Geometry check sheet. Reference: the model listing, model coordinates, mm. A direction names the side the tool comes from. Coordinates: 2 decimals unless noted, no trailing zeros. Write each loop counter-clockwise with the first axis right and the second up, starting at its lowest first coordinate (ties: lowest second). Pieces come first, ordered by that corner, then holes.
from build123d import *

# Parameters (mm, degrees)
SKETCH1_W           = 29
SKETCH1_H           = 15.5
BOSS_EXTRUDE1_DEPTH = 8
SHELL1_T            = -1
SKETCH2_W           = 1
SKETCH2_H           = 13.5
BOSS_EXTRUDE2_DEPTH = 7
SKETCH3_W           = 8
SKETCH3_H           = 3
CUT_EXTRUDE1_DEPTH  = 7


with BuildPart() as part:
    # Sketch1 → Boss-Extrude1 (new body)
    with BuildSketch(Plane(origin=(0, 0, 0), x_dir=(1, 0, 0), z_dir=(0, 1, 0))):
        Rectangle(SKETCH1_W, SKETCH1_H)
    extrude(amount=BOSS_EXTRUDE1_DEPTH)

    # Shell1
    shell1_openings = [part.faces().sort_by_distance(p)[0] for p in [
        (0, 8, 0),
    ]]
    offset(amount=SHELL1_T, openings=shell1_openings, kind=Kind.INTERSECTION)

    # Sketch2 → Boss-Extrude2 (add)
    with BuildSketch(Plane(origin=(0, 1, 0), x_dir=(1, 0, 0), z_dir=(0, 1, 0))):
        Rectangle(SKETCH2_W, SKETCH2_H)
    extrude(amount=BOSS_EXTRUDE2_DEPTH)

    # Sketch3 → Cut-Extrude1 (cut)
    with BuildSketch(Plane(origin=(0, 1, 0), x_dir=(1, 0, 0), z_dir=(0, 1, 0))):
        with Locations((-7.25, 5.25)):
            Rectangle(SKETCH3_W, SKETCH3_H)
        with Locations((7.25, 5.25)):
            Rectangle(SKETCH3_W, SKETCH3_H)
        with Locations((7.25, -5.25)):
            Rectangle(SKETCH3_W, SKETCH3_H)
        with Locations((-7.25, -5.25)):
            Rectangle(SKETCH3_W, SKETCH3_H)
    extrude(amount=-CUT_EXTRUDE1_DEPTH, mode=Mode.SUBTRACT)


solid = part.part
1. Sectioned sample at A-A, the plane x = -9.5. Record the boundary of the cut face in (y, z), and give its area (3 significant figures).
Computed values:
outline: (0, -7.75) - (8, -7.75) - (8, -6.75) - (0, -6.75) - close; (0, -3.75) - (1, -3.75) - (1, 3.75) - (0, 3.75) - close; (0, 6.75) - (8, 6.75) - (8, 7.75) - (0, 7.75) - close
area: 23.5 mm2
2. Thickness scan on line 1 along X through (y, z) = (5.75, -3.5); line 2 along Z through (x, y) = (8.5, 0.5); line 3 along Z through (x, y) = (-5, 5.5). Record the ranges inside material, lowest first.
Computed values:
line 1: x = -14.5 to -13.5, -0.5 to 0.5, 13.5 to 14.5
line 2: z = -7.75 to -6.75, -3.75 to 3.75, 6.75 to 7.75
line 3: z = -7.75 to -6.75, 6.75 to 7.75
3. Sectioned sample at B-B, the plane z = 5.75. Record the boundary of the cut face in (x, y).
Computed values:
outline: (-14.5, 0) - (-11.25, 0) - (-11.25, 1) - (-13.5, 1) - (-13.5, 8) - (-14.5, 8) - close; (-3.25, 0) - (3.25, 0) - (3.25, 1) - (0.5, 1) - (0.5, 8) - (-0.5, 8) - (-0.5, 1) - (-3.25, 1) - close; (11.25, 0) - (14.5, 0) - (14.5, 8) - (13.5, 8) - (13.5, 1) - (11.25, 1) - close
4. Draft check along Z on faces 4 (the flat face through (0, 8, 0)), 5 (the flat face through (0, 4, -7.75)), 6 (the flat face through (-11.25, 0.5, 5.3)). Enter one of: released by +Z, released by -Z, zero draft, split by the parting line, or undercut.
Computed values:
face 4: zero draft
face 5: released by -Z
face 6: undercut
5. Sectioned sample at D-D, the plane z = -1.75. Record the boundary of the cut face in (x, y).
Computed values:
outline: (-14.5, 0) - (14.5, 0) - (14.5, 8) - (13.5, 8) - (13.5, 1) - (0.5, 1) - (0.5, 8) - (-0.5, 8) - (-0.5, 1) - (-13.5, 1) - (-13.5, 8) - (-14.5, 8) - close
6. Access from +Z, -Z, +X, -X, +Y, -Y to the whole of each face (thin tool, end or side, straight path). Record for faces 1 (the flat face through (-0.5, 4, 0)), 2 (the flat face through (3.25, 0.5, 5.3)), 3 (the flat face through (-14.5, 4, 0)).
Computed values:
face 1: +Y
face 2: +Y, -Y
face 3: +Z, -Z, -X, +Y, -Y
7. Gauge pin test, flat end, axial feed: pin 1 Ø4 at (x, z) = (-10, 3.5) entering from +Y. Record the tip position at first contact, or that the pin passes through.
Computed values:
pin 1: stops at y = 1
8. Sectioned sample at C-C, the plane y = 2.75. Record the boundary of the cut face in (x, z), and give its area (3 significant figures).
Computed values:
outline: (-14.5, -7.75) - (14.5, -7.75) - (14.5, 7.75) - (-14.5, 7.75) - close; hole (-13.5, -6.75) - (-0.5, -6.75) - (-0.5, 6.75) - (-13.5, 6.75) - close; hole (0.5, -6.75) - (13.5, -6.75) - (13.5, 6.75) - (0.5, 6.75) - close
area: 98.5 mm2
